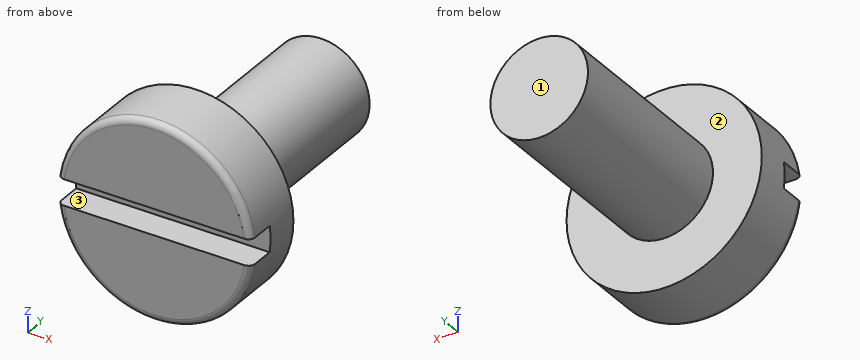
Solid Edge part; units mm, degrees
sketch "Sketch1" plane through (0, 0, 0) normal (0, -1, 0) x (1, 0, 0)
  circle A0 centre (0, 0) radius 1.5
extrude "Protrusion1" add sketch "Sketch1" against normal blind 6
sketch "Sketch2" plane through (0, 0, 0) normal (0, -1, 0) x (1, 0, 0)
  circle A0 centre (0, 0) radius 3
extrude "ExtrudedProtrusion_2" add sketch "Sketch2" along normal blind 2
cosmetic_thread "Thread1"
sketch "Sketch3" plane through (0, -2, 0) normal (0, -1, 0) x (1, 0, 0)
  line L0 (2.9734, -0.3984) -> (-2.9734, -0.3984)
  line L1 (-2.9734, 0.3984) -> (2.9734, 0.3984)
  arc A0 (2.9734, 0.3984) -> (2.9734, -0.3984) centre (0, 0) cw
  arc A1 (-2.9734, -0.3984) -> (-2.9734, 0.3984) centre (0, 0) cw
extrude "ExtrudedCutout_1" cut sketch "Sketch3" against normal blind 0.9
fillet "Round_1" radius 0.2 2 edges at (0, -2, -3) (0, -2, 3)
properties material "Nylon, general purpose"
Input: part model. Units: mm. Frame: model coordinates. Face numbers are marked on the shaded views. A direction names the side the tool comes from. Coordinates: 2 decimals unless noted, no trailing zeros. Loops run counter-clockwise (first coordinate to the right, second up) from the corner with the lowest first, then second, coordinate; pieces in that order, holes last. Notation, with made-up numbers: (52, -5) - (57, -5) arc R8 cw to (57, 5) - close; hole circle Ø11 at (-12.5, 59.5). An arc over 180 degrees is marked (long way). Answer in a Markdown table with one row per item.
(1) Cut plane C-C on y = 5.25. Output: boundary loops of the cut face in (x, z), plus the area to 3 significant figures.
Model answer:
| item | result |
|---|---|
| outline | circle Ø3 at (0, 0) |
| area | 7.07 mm² |
(2) Cut plane B-B on z = 0. Output: boundary loops of the cut face in (x, y).
Model answer:
| item | result |
|---|---|
| outline | (-3, -1.1) - (3, -1.1) - (3, 0) - (1.5, 0) - (1.5, 6) - (-1.5, 6) - (-1.5, 0) - (-3, 0) - close |
(3) Cut plane D-D on y = -0.25. Output: boundary loops of the cut face in (x, z), plus the area to 3 significant figures.
Model answer:
| item | result |
|---|---|
| outline | circle Ø6 at (0, 0) |
| area | 28.3 mm² |
(4) Material intervals for L1, parallel to Y at x = -2.1, z = -1.5; L2, parallel to X at y = 5, z = -1; L3, parallel to Z at x = 1.7, y = -1, sorted ascending. Write a range as from..to.
Model answer:
| item | result |
|---|---|
| L1 | y = -2..0 |
| L2 | x = -1.12..1.12 |
| L3 | z = -2.47..2.47 |
(5) Set-up query: the marked faces 1, 2 and 3. Return all of +Z, -Z, +X, -X, +Y, -Y with unobstructed straight access to the full face (end or side cutting, diameter ignored); none if empty.
Model answer:
| item | result |
|---|---|
| face 1 | +Z, -Z, +X, -X, +Y |
| face 2 | +Y |
| face 3 | +X, -X, -Y |
(6) Pin query (flat end, axial travel): P1, Ø1, axis at y = -0.5, z = -2, coming from the -X side; P2, Ø3, axis at x = -1.5, z = -0.5, coming from the +Y side; P3, Ø0.6, axis at x = 0.5, z = 0, coming from the -Y side; P4, Ø2, axis at y = -0.5, z = -2, coming from the -X side. Return the tip coordinate at first contact, or that it passes through.
Model answer:
| item | result |
|---|---|
| P1 | stops at x = -2.6 |
| P2 | stops at y = 6 |
| P3 | stops at y = -1.1 |
| P4 | stops at x = -2.83 |
(7) Cut plane A-A on x = 0. Output: boundary loops of the cut face in (y, z), plus the area to 3 significant figures.
Model answer:
| item | result |
|---|---|
| outline | (-2, -2.8) arc R0.2 ccw to (-1.8, -3) - (0, -3) - (0, -1.5) - (6, -1.5) - (6, 1.5) - (0, 1.5) - (0, 3) - (-1.8, 3) arc R0.2 ccw to (-2, 2.8) - (-2, 0.4) - (-1.1, 0.4) - (-1.1, -0.4) - (-2, -0.4) - close |
| area | 29.3 mm² |
